Job drawing, mm, ordinate dimensions from the low corner. One solid piece. A direction names the side the tool comes from. Round coordinates to 2 decimals unless told otherwise and drop trailing zeros. Loops run counter-clockwise (first coordinate to the right, second up) from the corner with the lowest first, then second, coordinate; pieces in that order, holes last.
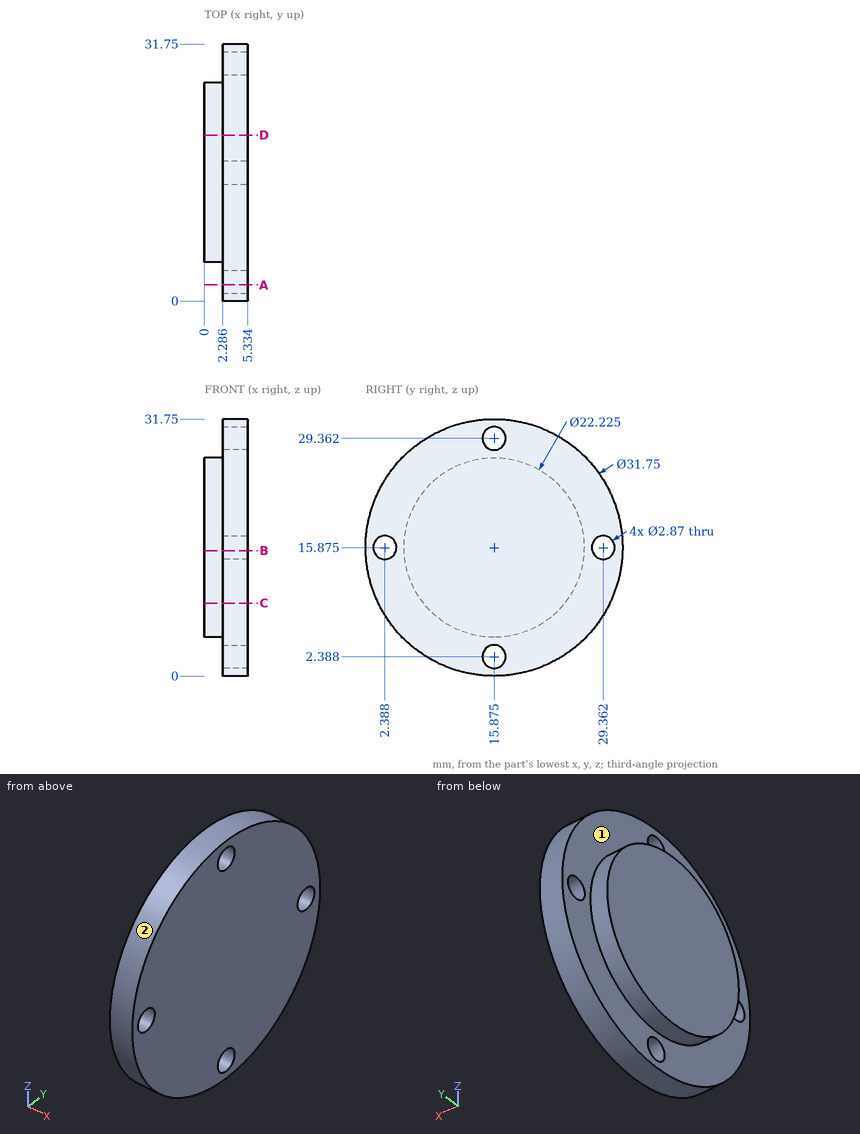
Item 1: 3-axis set-ups, long thin cutter, end or side, ignore diameter. For the marked faces 1 and 2: which of +Z, -Z, +X, -X, +Y, -Y reach the whole face in a straight line?
Answers follow:
face 1: -X
face 2: +X, -X
Item 2: Probe line 1 (Z direction, x = 5.1, y = 16); line 2 (X direction, y = 11, z = 30); line 3 (Z direction, x = 3.45, y = 15.5) (1 decimal). List the from-to ranges inside material, lowest first.
Answers follow:
line 1: z = 0 to 0.96, 3.82 to 27.93, 30.79 to 31.75
line 2: x = 2.29 to 5.33
line 3: z = 0 to 1, 3.8 to 28, 30.7 to 31.7
Item 3: Cut at A-A, the plane y = 2. Give the cut face in (x, z), plus the area to 3 significant figures.
Answers follow:
outline: (2.29, 8.16) - (5.33, 8.16) - (5.33, 14.49) - (2.29, 14.49) - close; (2.29, 17.26) - (5.33, 17.26) - (5.33, 23.59) - (2.29, 23.59) - close
area: 38.6 mm2
Item 4: Cut at C-C, the plane z = 9. Give the cut face in (x, y) (1 decimal).
Answers follow:
outline: (0, 7.1) - (2.3, 7.1) - (2.3, 1.6) - (5.3, 1.6) - (5.3, 30.2) - (2.3, 30.2) - (2.3, 24.6) - (0, 24.6) - close
Item 5: Cut at D-D, the plane y = 20.5. Give the cut face in (x, z), plus the area to 3 significant figures.
Answers follow:
outline: (0, 5.77) - (2.29, 5.77) - (2.29, 0.69) - (5.33, 0.69) - (5.33, 31.06) - (2.29, 31.06) - (2.29, 25.98) - (0, 25.98) - close
area: 139 mm2
Item 6: Cut at B-B, the plane z = 15.5. Give the cut face in (x, y) (1 decimal).
Answers follow:
outline: (0, 4.8) - (2.3, 4.8) - (2.3, 3.8) - (5.3, 3.8) - (5.3, 28) - (2.3, 28) - (2.3, 27) - (0, 27) - close; (2.3, 0) - (5.3, 0) - (5.3, 1) - (2.3, 1) - close; (2.3, 30.7) - (5.3, 30.7) - (5.3, 31.7) - (2.3, 31.7) - close
Item 7: Flat gauge pins, fed straight in: P1, Ø2.5, axis at y = 15.88, z = 29.36, coming from the -X side; P2, Ø1.5, axis at x = 1.5, y = 14, coming from the +Z side. Where does each tip first touch, or does it go through?
Answers follow:
P1: passes through
P2: stops at z = 26.93
